```python
from build123d import *

# Parameters (mm, degrees)
SKETCH1_W           = 17
SKETCH1_H           = 20
BOSS_EXTRUDE1_DEPTH = 3
SKETCH2_W           = 17
SKETCH2_H           = 3
BOSS_EXTRUDE2_DEPTH = 17
RIB1_REACH          = 30.089
SKETCH3_WALL_W      = 82.219918182
SKETCH3_WALL_H      = 2
RIB4_REACH          = 30.089
SKETCH4_WALL_W      = 82.219918182
SKETCH4_WALL_H      = 2
CUT_EXTRUDE1_DEPTH  = 17
CUT_EXTRUDE2_DEPTH  = 17
BOSS_EXTRUDE3_DEPTH = 1
BOSS_EXTRUDE4_DEPTH = 1
FILLET1_R           = 0.2


with BuildPart() as part:
    # Sketch1 → Boss-Extrude1 (new body)
    with BuildSketch(Plane(origin=(0, 0, 0), x_dir=(1, 0, 0), z_dir=(0, 1, 0))):
        Rectangle(SKETCH1_W, SKETCH1_H)
    extrude(amount=BOSS_EXTRUDE1_DEPTH)

    # Sketch2 → Boss-Extrude2 (add)
    with BuildSketch(Plane(origin=(0, 3, 0), x_dir=(1, 0, 0), z_dir=(0, 1, 0))):
        with Locations((0, -8.5)):
            Rectangle(SKETCH2_W, SKETCH2_H)
    extrude(amount=BOSS_EXTRUDE2_DEPTH)

    # Sketch3 wall → Rib1 (add, up to next)
    with BuildSketch(Plane(origin=(8.5, 11.5, -1.5), x_dir=(0, -0.707106781187, -0.707106781187), z_dir=(0, 0.707106781187, -0.707106781187)), mode=Mode.PRIVATE) as rib1_sk1:
        with Locations((0, 1)):
            Rectangle(SKETCH3_WALL_W, SKETCH3_WALL_H)
    rib1_tool1 = extrude(rib1_sk1.sketch, amount=-RIB1_REACH, mode=Mode.PRIVATE) - part.part
    add(rib1_tool1.solids().sort_by_distance((8.5, 11.5, -1.5))[0])

    # Sketch4 wall → Rib4 (add, up to next)
    with BuildSketch(Plane(origin=(-8.5, 11.5, -1.5), x_dir=(0, -0.707106781187, -0.707106781187), z_dir=(0, -0.707106781187, 0.707106781187)), mode=Mode.PRIVATE) as rib4_sk1:
        with Locations((0, 1)):
            Rectangle(SKETCH4_WALL_W, SKETCH4_WALL_H)
    rib4_tool1 = extrude(rib4_sk1.sketch, amount=RIB4_REACH, mode=Mode.PRIVATE) - part.part
    add(rib4_tool1.solids().sort_by_distance((-8.5, 11.5, -1.5))[0])

    # Sketch5 → Cut-Extrude1 (cut)
    with BuildSketch(Plane.XY.offset(10)):
        with BuildLine():
            Line((-0.5, 5.5), (0.5, 5.5))
            ThreePointArc((0.5, 5.5), (2.267766953, 6.232233047), (3, 8))
            Line((3, 8), (3, 12))
            ThreePointArc((3, 12), (2.267766953, 13.767766953), (0.5, 14.5))
            Line((0.5, 14.5), (-0.5, 14.5))
            ThreePointArc((-0.5, 14.5), (-2.267766953, 13.767766953), (-3, 12))
            Line((-3, 12), (-3, 8))
            ThreePointArc((-3, 8), (-2.267766953, 6.232233047), (-0.5, 5.5))
        make_face()
    extrude(amount=-CUT_EXTRUDE1_DEPTH, mode=Mode.SUBTRACT)

    # Sketch6 → Cut-Extrude2 (cut)
    with BuildSketch(Plane.XZ):
        with BuildLine():
            Line((-0.5, 4.5), (0.5, 4.5))
            ThreePointArc((0.5, 4.5), (2.267766953, 3.767766953), (3, 2))
            Line((3, 2), (3, -2))
            ThreePointArc((3, -2), (2.267766953, -3.767766953), (0.5, -4.5))
            Line((0.5, -4.5), (-0.5, -4.5))
            ThreePointArc((-0.5, -4.5), (-2.267766953, -3.767766953), (-3, -2))
            Line((-3, -2), (-3, 2))
            ThreePointArc((-3, 2), (-2.267766953, 3.767766953), (-0.5, 4.5))
        make_face()
    extrude(amount=-CUT_EXTRUDE2_DEPTH, mode=Mode.SUBTRACT)

    # Sketch7 → Boss-Extrude3 (add)
    with BuildSketch(Plane.XZ):
        with BuildLine():
            Line((1.5, 8), (-1.5, 8))
            ThreePointArc((-1.5, 8), (-1.853553391, 7.853553391), (-2, 7.5))
            Line((-2, 7.5), (-2, 6.5))
            ThreePointArc((-2, 6.5), (-1.853553391, 6.146446609), (-1.5, 6))
            Line((-1.5, 6), (1.5, 6))
            ThreePointArc((1.5, 6), (1.853553391, 6.146446609), (2, 6.5))
            Line((2, 6.5), (2, 7.5))
            ThreePointArc((2, 7.5), (1.853553391, 7.853553391), (1.5, 8))
        make_face()
        with BuildLine():
            Line((-2, -7.5), (-2, -6.5))
            ThreePointArc((-2, -6.5), (-1.853553391, -6.146446609), (-1.5, -6))
            Line((-1.5, -6), (1.5, -6))
            ThreePointArc((1.5, -6), (1.853553391, -6.146446609), (2, -6.5))
            Line((2, -6.5), (2, -7.5))
            ThreePointArc((2, -7.5), (1.853553391, -7.853553391), (1.5, -8))
            Line((1.5, -8), (-1.5, -8))
            ThreePointArc((-1.5, -8), (-1.853553391, -7.853553391), (-2, -7.5))
        make_face()
    extrude(amount=BOSS_EXTRUDE3_DEPTH)

    # Sketch8 → Boss-Extrude4 (add)
    with BuildSketch(Plane.XY.offset(10)):
        with BuildLine():
            Line((-1.5, 4), (1.5, 4))
            ThreePointArc((1.5, 4), (1.853553391, 3.853553391), (2, 3.5))
            Line((2, 3.5), (2, 2.5))
            ThreePointArc((2, 2.5), (1.853553391, 2.146446609), (1.5, 2))
            Line((1.5, 2), (-1.5, 2))
            ThreePointArc((-1.5, 2), (-1.853553391, 2.146446609), (-2, 2.5))
            Line((-2, 2.5), (-2, 3.5))
            ThreePointArc((-2, 3.5), (-1.853553391, 3.853553391), (-1.5, 4))
        make_face()
        with BuildLine():
            Line((2, 16.5), (2, 17.5))
            ThreePointArc((2, 17.5), (1.853553391, 17.853553391), (1.5, 18))
            Line((1.5, 18), (-1.5, 18))
            ThreePointArc((-1.5, 18), (-1.853553391, 17.853553391), (-2, 17.5))
            Line((-2, 17.5), (-2, 16.5))
            ThreePointArc((-2, 16.5), (-1.853553391, 16.146446609), (-1.5, 16))
            Line((-1.5, 16), (1.5, 16))
            ThreePointArc((1.5, 16), (1.853553391, 16.146446609), (2, 16.5))
        make_face()
    extrude(amount=BOSS_EXTRUDE4_DEPTH)

    # Fillet1
    fillet1_edges = [part.edges().sort_by_distance(p)[0] for p in [
        (-1.853553391, -1, 7.853553391),
        (-2, -1, 7),
        (-1.853553391, -1, 6.146446609),
        (0, -1, 6),
        (1.853553391, -1, 6.146446609),
        (2, -1, 7),
        (1.853553391, -1, 7.853553391),
        (0, -1, 8),
        (1.853553391, -1, -7.853553391),
        (2, -1, -7),
        (1.853553391, -1, -6.146446609),
        (0, -1, -6),
        (-1.853553391, -1, -6.146446609),
        (-2, -1, -7),
        (-1.853553391, -1, -7.853553391),
        (0, -1, -8),
        (-1.853553391, 3.853553391, 11),
        (-2, 3, 11),
        (-1.853553391, 2.146446609, 11),
        (0, 2, 11),
        (1.853553391, 2.146446609, 11),
        (2, 3, 11),
        (1.853553391, 3.853553391, 11),
        (0, 4, 11),
        (1.853553391, 16.146446609, 11),
        (2, 17, 11),
        (1.853553391, 17.853553391, 11),
        (0, 18, 11),
        (-1.853553391, 17.853553391, 11),
        (-2, 17, 11),
        (-1.853553391, 16.146446609, 11),
        (0, 16, 11),
    ]]
    fillet(fillet1_edges, radius=FILLET1_R)


solid = part.part
```
Here's how the part is built. I have some questions about the finished solid (model axes, mm). A direction names the side the tool comes from. Give positions to 0.01 mm unless a question says otherwise; leave off trailing zeros. Order: outer loops, then holes, each group sorted by start corner. A loop starts at its lowest first (then second) coordinate and runs counter-clockwise, first axis right, second up. Notation, with made-up numbers: (43, 5) -> (101, 5) arc R28 ccw to (101, 32) -> close; hole circle Ø11 at (30.25, 63). An arc over 180 degrees is marked (long way). Use CSV: the item, a comma, the result in double quotes. Start each with the question number.
Item 1: On a 3-axis mill with a long thin cutter (end or side, diameter ignored), from which of +Z, -Z, +X, -X, +Y, -Y can I reach the whole of each face in a straight line? I mean faces 4 (the cylindrical face through (-2, 1, -4)), 5 (the flat face through (0, 20, 8)), 6 (the flat face through (-3, 10, 9)), 7 (the flat face through (0, 17, 11)), 8 (the flat face through (0, 4, 10.4)). Say none if no direction works.
Item 2: Thinking about a two-plate mould opening in X: for faces 1 (the cylindrical face through (-2, 14, 9)), 2 (the flat face through (-2, 17, 10.4)), 3 (the flat face through (-4, 10, 10)), which applies, pulls with the +X half, pulls with the -X half, needs draft (parallel to the pull), parting line crosses it, or undercut?
Item 3: I'm going to push flat-ended pins straight in: P1, Ø2, axis at x = 2, z = -6, coming from the -Y side; P2, Ø6, axis at x = -0.5, z = -3, coming from the +Y side; P3, Ø0.6, axis at x = 0.5, y = -0.5, coming from the +Z side; P4, Ø0.9, axis at y = 3, z = 10.5, coming from the -X side. Where does each tip first touch, or does it pass through?
Item 4: Suppose I cut it at A-A (y = 11). List the corners of the cut face in (x, z) for me.
Item 5: If I drill on probe 1 along X at (y, z) = (12.5, 4); probe 2 along Z at (x, y) = (0.5, 2.5); probe 3 along X at (y, z) = (2.75, -4), over which ranges is the centre line in solid material (lowest first)? Write a range as [from, to].
Item 6: Suppose I cut it at D-D (y = 17). List the corners of the cut face in (x, z) for me.
Item 7: Suppose I cut it at C-C (z = -5.25). List the corners of the cut face in (x, y) for me, and give its area (3 significant figures).
Item 8: Suppose I cut it at B-B (z = -0.5). List the corners of the cut face in (x, y) for me, and give its area (3 significant figures).
Answer block:
1,face 4,"+Y, -Y"
1,face 5,"+Z, -Z, +X, -X, +Y"
1,face 6,"+Z, -Z"
1,face 7,"+Z, +X, -X, +Y, -Y"
1,face 8,"+Z, +X, -X"
2,face 1,"undercut"
2,face 2,"pulls with the -X half"
2,face 3,"needs draft"
3,P1,"stops at y = -1"
3,P2,"stops at y = 3"
3,P3,"stops at z = 8"
3,P4,"stops at x = -2"
4,outline,"(-8.5, -2) -> (-6.5, -2) -> (-6.5, 7) -> (-3, 7) -> (-3, 10) -> (-8.5, 10) -> close; (3, 7) -> (6.5, 7) -> (6.5, -2) -> (8.5, -2) -> (8.5, 10) -> (3, 10) -> close"
5,probe 1,"x = [-8.5, -6.5], [6.5, 8.5]"
5,probe 2,"z = [-10, -4.5], [4.5, 11]"
5,probe 3,"x = [-8.5, -2], [2, 8.5]"
6,outline,"(-8.5, 4) -> (-6.5, 4) -> (-6.5, 7) -> (6.5, 7) -> (6.5, 4) -> (8.5, 4) -> (8.5, 10) -> (2, 10) -> (2, 10.8) arc R0.2 ccw to (1.8, 11) -> (-1.8, 11) arc R0.2 ccw to (-2, 10.8) -> (-2, 10) -> (-8.5, 10) -> close"
7,outline,"(-8.5, 0) -> (8.5, 0) -> (8.5, 7.75) -> (6.5, 7.75) -> (6.5, 3) -> (-6.5, 3) -> (-6.5, 7.75) -> (-8.5, 7.75) -> close"
7,area,"70.0 mm^2"
8,outline,"(-8.5, 0) -> (-3, 0) -> (-3, 3) -> (-6.5, 3) -> (-6.5, 12.5) -> (-8.5, 12.5) -> close; (3, 0) -> (8.5, 0) -> (8.5, 12.5) -> (6.5, 12.5) -> (6.5, 3) -> (3, 3) -> close"
8,area,"71.0 mm^2"
